CAD build for the part. Positions are in the model's coordinates, mm. Face numbers are marked on the shaded views. Round coordinates to 2 decimals unless told otherwise and drop trailing zeros. Loops run counter-clockwise (first coordinate to the right, second up) from the corner with the lowest first, then second, coordinate; pieces in that order, holes last. Notation, with made-up numbers: (27.5, -9) - (45.5, -9) arc R15 cw to (45.5, 6) - close; hole circle Ø9 at (7.5, 40). An arc over 180 degrees is marked (long way). Use one line per item in the form item = value.
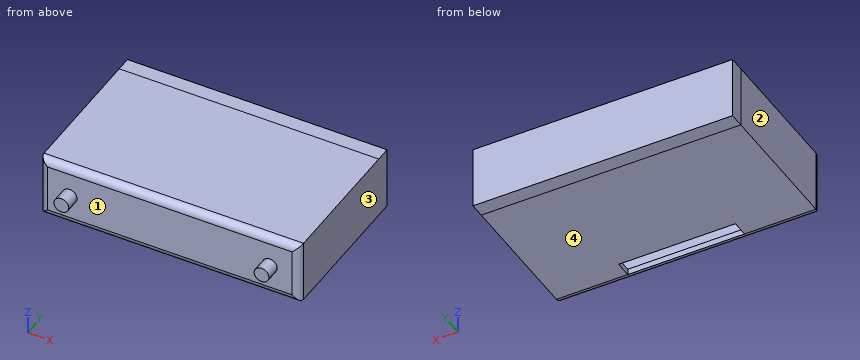
from build123d import *

# Parameters (mm, degrees)
SKETCH1_W           = 175
SKETCH1_H           = 42.3
BOSS_EXTRUDE1_DEPTH = 4
SKETCH1_3_W         = 175
SKETCH1_3_H         = 42.3
SKETCH1_3_W_2       = 167
SKETCH1_3_H_2       = 34.3
BOSS_EXTRUDE2_DEPTH = 96
SKETCH1_4_R         = 5
BOSS_EXTRUDE3_DEPTH = 10
FILLET1_R           = 5
SKETCH3_W           = 78.73
SKETCH3_H           = 11.03
CUT_EXTRUDE1_DEPTH  = 4
SKETCH4_W           = 174.998654926
SKETCH4_H           = 42.297309852
BOSS_EXTRUDE4_DEPTH = 10


with BuildPart() as part:
    # Sketch1 → Boss-Extrude1 (new body)
    with BuildSketch(Plane(origin=(0, 0, 0), x_dir=(1, 0, 0), z_dir=(0, 1, 0))):
        with Locations((35.322931561, 0)):
            Rectangle(SKETCH1_W, SKETCH1_H)
    extrude(amount=BOSS_EXTRUDE1_DEPTH)

    # Sketch1_3 → Boss-Extrude2 (add)
    with BuildSketch(Plane(origin=(0, 0, 0), x_dir=(1, 0, 0), z_dir=(0, 1, 0))):
        with Locations((35.322931561, 0)):
            Rectangle(SKETCH1_3_W, SKETCH1_3_H)
        with Locations((35.322931561, 0)):
            Rectangle(SKETCH1_3_W_2, SKETCH1_3_H_2, mode=Mode.SUBTRACT)
    extrude(amount=BOSS_EXTRUDE2_DEPTH)

    # Sketch1_4 → Boss-Extrude3 (add)
    with BuildSketch(Plane(origin=(0, 0, 0), x_dir=(1, 0, 0), z_dir=(0, 1, 0))):
        with Locations(Location((-32.177068439, 0, 0), (0, 0, 270))):
            Circle(SKETCH1_4_R)
        with Locations(Location((102.822931561, 0, 0), (0, 0, 270))):
            Circle(SKETCH1_4_R)
    extrude(amount=-BOSS_EXTRUDE3_DEPTH)

    # Fillet1
    fillet1_edges = [part.edges().sort_by_distance(p)[0] for p in [
        (-52.177068439, 0, 0),
        (35.322931561, 0, -21.15),
        (122.822931561, 0, 0),
        (35.322931561, 0, 21.15),
    ]]
    fillet(fillet1_edges, radius=FILLET1_R)

    # Sketch3 → Cut-Extrude1 (cut)
    with BuildSketch(Plane(origin=(0, 0, -21.15), x_dir=(-1, 0, 0), z_dir=(0, 0, -1))):
        with Locations((-35.322931561, 10.515)):
            Rectangle(SKETCH3_W, SKETCH3_H)
    extrude(amount=-CUT_EXTRUDE1_DEPTH, mode=Mode.SUBTRACT)

    # Sketch4 → Boss-Extrude4 (add)
    with BuildSketch(Plane(origin=(0, 96, 0), x_dir=(1, 0, 0), z_dir=(0, 1, 0))):
        with Locations((35.323604098, 0)):
            Rectangle(SKETCH4_W, SKETCH4_H)
    extrude(amount=BOSS_EXTRUDE4_DEPTH)


solid = part.part
1) Slice it at B-B (y = 38.5). Write the cut outline in (x, z), plus the area to 3 significant figures.
Report:
outline = (-52.18, -21.15) - (122.82, -21.15) - (122.82, 21.15) - (-52.18, 21.15) - close; hole (-48.18, -17.15) - (118.82, -17.15) - (118.82, 17.15) - (-48.18, 17.15) - close
area = 1,670 mm^2
2) Flat gauge pins, fed straight in: pin 1 (1.2 mm diameter, centred on x = 42.5, z = -20, fed in from -Y); pin 2 (2 mm diameter, centred on x = 6.5, z = 4.5, fed in from -Y). Where does each tip first touch, or does it go through?
Report:
pin_1 = 1.2
pin_2 = 0
3) Drill centre lines: probe 1 along X at (y, z) = (51, -3); probe 2 along Y at (x, z) = (-0.5, -8); probe 3 along Z at (x, y) = (-8, 69.5). Where is each one in solid material? Low to high.
Report:
probe_1 = -52.18 to -48.18, 118.82 to 122.82
probe_2 = 0 to 4, 96 to 106
probe_3 = -21.15 to -17.15, 17.15 to 21.15
4) Two-plate mould, pull along X, no slides. Class the marked faces 1, 2, 3 and 4: +X half, -X half, draft (parallel to the pull), parting line (faces both ways), or undercut.
Report:
face_1 = undercut
face_2 = -X half
face_3 = +X half
face_4 = draft
